```python
from build123d import *

# Parameters (mm, degrees)
SKETCH1_W           = 190
SKETCH1_H           = 114
BOSS_EXTRUDE1_DEPTH = 2.5
SKETCH3_W           = 70
SKETCH3_H           = 23
CUT_EXTRUDE2_DEPTH  = 10
SKETCH4_R           = 2
CUT_EXTRUDE3_DEPTH  = 10


with BuildPart() as part:
    # Sketch1 → Boss-Extrude1 (new body)
    with BuildSketch(Plane.XY):
        Rectangle(SKETCH1_W, SKETCH1_H)
    extrude(amount=BOSS_EXTRUDE1_DEPTH)

    # Sketch3 → Cut-Extrude2 (cut)
    with BuildSketch(Plane.XY.offset(2.5)):
        with Locations((-4, -36.5)):
            Rectangle(SKETCH3_W, SKETCH3_H)
    extrude(amount=-CUT_EXTRUDE2_DEPTH, mode=Mode.SUBTRACT)

    # Sketch4 → Cut-Extrude3 (cut)
    with BuildSketch(Plane.XY.offset(2.5)):
        with Locations((-90, 52)):
            Circle(SKETCH4_R)
        with Locations(Location((90, 52, 0), (0, 0, 180))):
            Circle(SKETCH4_R)
        with Locations((-90, -52)):
            Circle(SKETCH4_R)
        with Locations(Location((90, -52, 0), (0, 0, 180))):
            Circle(SKETCH4_R)
    extrude(amount=-CUT_EXTRUDE3_DEPTH, mode=Mode.SUBTRACT)


solid = part.part
```
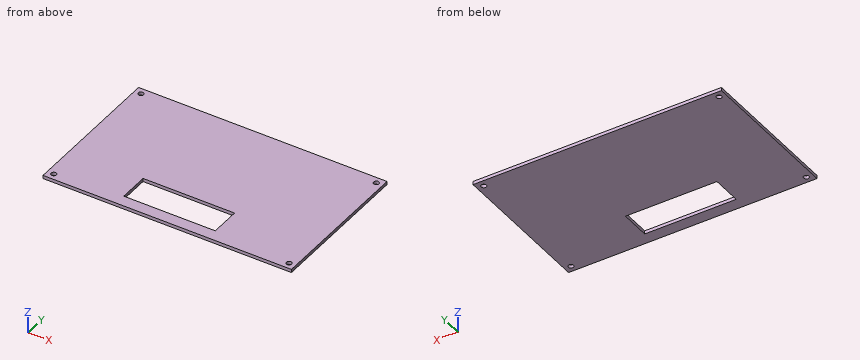
CAD build for the part. Positions are in the model's coordinates, mm. Give positions to 0.01 mm unless a question says otherwise; leave off trailing zeros. Order: outer loops, then holes, each group sorted by start corner. A loop starts at its lowest first (then second) coordinate and runs counter-clockwise, first axis right, second up. Notation, with made-up numbers: M 47,48 L 55,48 A27 cw 55,82 Z; hole C -31,73 d9. An arc over 180 degrees is marked long. Put each result on its own line as item: value. Start each with the question number.
(1) Saw through at D-D, the plane x = -90. Write the cut outline in (y, z), then the cut area to 3 significant figures.
(2) Drill centre lines: line 1 along Y through (x, z) = (-90, 1.9); line 2 along X through (y, z) = (-27, 0.4); line 3 along Y through (x, z) = (-32.5, 2.1). Where is each one in solid material? Low to high.
(3) Saw through at A-A, the plane x = 16.5. Write the cut outline in (y, z), then the cut area to 4 significant figures.
(4) Flat gauge pin, fed straight in: pin 1 Ø5 at (x, y) = (-90, -52) entering from -Z. Where does the tip first touch, or does it go through?
(5) Saw through at B-B, the plane y = 52. Write the cut outline in (x, z).
(6) Saw through at C-C, the plane z = 0.55. Write the cut outline in (x, y), then the cut area to 3 significant figures.
Check result:
1. outline: M -57,0 L -54,0 L -54,2.5 L -57,2.5 Z; M -50,0 L 50,0 L 50,2.5 L -50,2.5 Z; M 54,0 L 57,0 L 57,2.5 L 54,2.5 Z
1. area: 265 mm2
2. line 1: y = -57 to -54, -50 to 50, 54 to 57
2. line 2: x = -95 to -39, 31 to 95
2. line 3: y = -57 to -48, -25 to 57
3. outline: M -57,0 L -48,0 L -48,2.5 L -57,2.5 Z; M -25,0 L 57,0 L 57,2.5 L -25,2.5 Z
3. area: 227.5 mm2
4. pin 1: stops at z = 0
5. outline: M -95,0 L -92,0 L -92,2.5 L -95,2.5 Z; M -88,0 L 88,0 L 88,2.5 L -88,2.5 Z; M 92,0 L 95,0 L 95,2.5 L 92,2.5 Z
6. outline: M -95,-57 L 95,-57 L 95,57 L -95,57 Z; hole C -90,-52 d4; hole C -90,52 d4; hole M -39,-48 L 31,-48 L 31,-25 L -39,-25 Z; hole C 90,-52 d4; hole C 90,52 d4
6. area: 20,000 mm2
